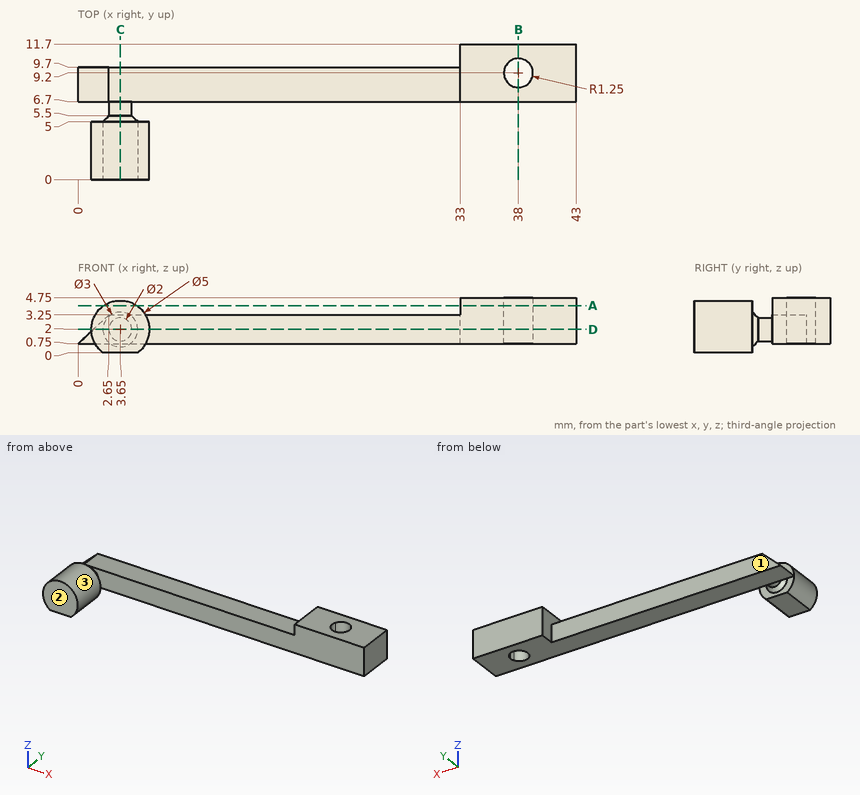
For this review, use the dimensioned drawing (mm, ordinates from the lowest corner) and the shaded views. A direction names the side the tool comes from. Give positions to 0.01 mm unless a question says otherwise; leave off trailing zeros. Order: outer loops, then holes, each group sorted by start corner. A loop starts at its lowest first (then second) coordinate and runs counter-clockwise, first axis right, second up. Notation, with made-up numbers: (-22, -12) - (35, -12) arc R11 ccw to (35, 1) - close; hole circle Ø10 at (27.25, -27.5). An arc over 180 degrees is marked (long way). Use CSV: the item, a comma, the result in double quotes. Start each with the question number.
Q1. Tool access review of the marked faces 1, 2 and 3: name each direction out of +Z, -Z, +X, -X, +Y, -Y from which nothing blocks a thin tool from reaching the whole face with its end or side.
Q2. Clearance check with flat-ended pins moving along their axes: pin 1 Ø1.2 at (x, z) = (16, 3) entering from -Y; pin 2 Ø3 at (x, y) = (18.5, 4) entering from -Z; pin 3 Ø2.5 at (x, y) = (12, 8) entering from -Z; pin 4 Ø2 at (y, z) = (8.5, 2) entering from -X (3 decimals). State where each tip first meets the part, or that it passes through.
Q3. To check wall thickness, follow line 1 along Y through (x, z) = (7.5, 2.6); line 2 along X through (y, z) = (8.25, 4); line 3 along X through (y, z) = (2.5, 1.8). State the ranges of each line that lie inside material, in increasing order. Write a range as [from, to].
Q4. We need section B-B, the plane x = 38. Write out the cut boundary in (y, z).
Q5. We need section D-D, the plane z = 2. Write out the cut boundary in (x, y) (3 decimals).
Q6. We need section A-A, the plane z = 4.05. Write out the cut boundary in (x, y).
Q7. We need section C-C, the plane x = 3.65. Write out the cut boundary in (y, z).
Outcome:
1,face 1,"+Z, -Z, -X, +Y"
1,face 2,"+Z, -Z, +X, -X, -Y"
1,face 3,"-Y"
2,pin 1,"stops at y = 6.7"
2,pin 2,"passes through"
2,pin 3,"stops at z = 0.75"
2,pin 4,"stops at x = 0.265"
3,line 1,"y = [6.7, 9.7]"
3,line 2,"x = [33, 37.19], [38.81, 43]"
3,line 3,"x = [1.16, 6.14]"
4,outline,"(6.7, 0.75) - (7.95, 0.75) - (7.95, 4.75) - (6.7, 4.75) - close; (10.45, 0.75) - (11.7, 0.75) - (11.7, 4.75) - (10.45, 4.75) - close"
5,outline,"(1.15, 0) - (6.15, 0) - (6.15, 5) - (5.15, 5) - (4.65, 5.5) - (4.65, 6.7) - (43, 6.7) - (43, 11.7) - (33, 11.7) - (33, 9.7) - (1.325, 9.7) - (1.325, 6.7) - (2.65, 6.7) - (2.65, 5.5) - (2.15, 5) - (1.15, 5) - close; hole circle Ø2.5 at (38, 9.2)"
6,outline,"(2.22, 0) - (5.08, 0) - (5.08, 5) - (2.22, 5) - close; (33, 6.7) - (43, 6.7) - (43, 11.7) - (33, 11.7) - close; hole circle Ø2.5 at (38, 9.2)"
7,outline,"(0, 0) - (5, 0) - (5, 0.5) - (5.5, 1) - (6.7, 1) - (6.7, 0.75) - (9.7, 0.75) - (9.7, 3.25) - (6.7, 3.25) - (6.7, 3) - (5.5, 3) - (5, 3.5) - (5, 4.5) - (0, 4.5) - close"
